CAD build for the part. Positions are in the model's coordinates, mm. Face numbers are marked on the shaded views. A direction names the side the tool comes from. Round coordinates to 2 decimals unless told otherwise and drop trailing zeros. Order: outer loops, then holes, each group sorted by start corner. A loop starts at its lowest first (then second) coordinate and runs counter-clockwise, first axis right, second up. Notation, with made-up numbers: M 31,7 L 48,7 A11 cw 48,14 Z; hole C -30,43.5 d7. An arc over 180 degrees is marked long. Answer as a JSON object with one key per item and string values.
```python
from build123d import *

# Parameters (mm, degrees)
CORTAR_EXTRUIR1_DEPTH = 9
CROQUIS5_R            = 4
CORTAR_EXTRUIR3_DEPTH = 27
CROQUIS6_R            = 2
CORTAR_EXTRUIR4_DEPTH = 10


with BuildPart() as part:
    # Croquis1 → Revolución1 (revolve)
    with BuildSketch(Plane(origin=(0, 0, 0), x_dir=(1, 0, 0), z_dir=(0, 1, 0))):
        Polygon((0, 1.5), (0, -9.5), (7, -9.5), (7, -13), (12.5, -13), (27.5, -13), (27.5, -7.5), (20, -7.5), (20, -2.5), (27.5, -2.5), (27.5, 2.5), (20, 2.5), (20, 7.5), (27.5, 7.5), (27.5, 13), (12.5, 13), (12.5, 6.5), (7.5, 1.5), align=None)
    revolve(axis=Axis((0, 0, 0), (0, 0, -1)))

    # Croquis2 → Cortar-Extruir1 (cut)
    with BuildSketch(Plane(origin=(0, 0, -1.5), x_dir=(-1, 0, 0), z_dir=(0, 0, -1))):
        Polygon((7.505553499, 0), (3.75277675, 6.5), (-3.75277675, 6.5), (-7.505553499, 0), (-3.75277675, -6.5), (3.75277675, -6.5), align=None)
    extrude(amount=-CORTAR_EXTRUIR1_DEPTH, mode=Mode.SUBTRACT)

    # Croquis5 → Cortar-Extruir3 (cut, through all)
    with BuildSketch(Plane.XY.offset(13)):
        with Locations((0, 24.5)):
            Circle(CROQUIS5_R)
        with Locations((12.25, 21.217622393)):
            Circle(CROQUIS5_R)
        with Locations((21.217622393, 12.25)):
            Circle(CROQUIS5_R)
        with Locations((24.5, 0)):
            Circle(CROQUIS5_R)
        with Locations((21.217622393, -12.25)):
            Circle(CROQUIS5_R)
        with Locations((12.25, -21.217622393)):
            Circle(CROQUIS5_R)
        with Locations((0, -24.5)):
            Circle(CROQUIS5_R)
        with Locations((-12.25, -21.217622393)):
            Circle(CROQUIS5_R)
        with Locations((-21.217622393, -12.25)):
            Circle(CROQUIS5_R)
        with Locations((-24.5, 0)):
            Circle(CROQUIS5_R)
        with Locations((-21.217622393, 12.25)):
            Circle(CROQUIS5_R)
        with Locations((-12.25, 21.217622393)):
            Circle(CROQUIS5_R)
    extrude(amount=-CORTAR_EXTRUIR3_DEPTH, mode=Mode.SUBTRACT)

    # Croquis6 → Cortar-Extruir4 (cut)
    with BuildSketch(Plane(origin=(0, 0, 7.5), x_dir=(-1, 0, 0), z_dir=(0, 0, -1))):
        Circle(CROQUIS6_R)
    extrude(amount=-CORTAR_EXTRUIR4_DEPTH, mode=Mode.SUBTRACT)


solid = part.part
```
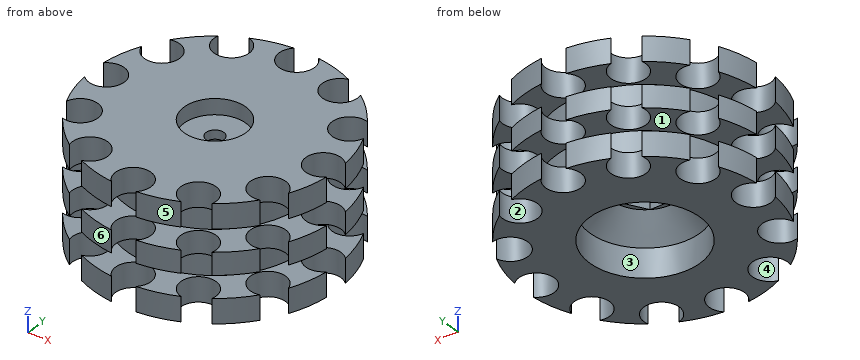
Item 1: Drop flat-ended pins along their axis: pin 1 Ø1.9 at (x, y) = (4.5, -2) entering from -Z; pin 2 Ø10 at (y, z) = (16.5, 5) entering from -X; pin 3 Ø6.5 at (x, y) = (-21.22, 12.25) entering from -Z; pin 4 Ø12 at (y, z) = (6.5, 5.5) entering from +X. Give the stop position or say it passes through.
Worked answers:
{"pin 1": "stops at z = 7.5", "pin 2": "stops at x = -22.29", "pin 3": "passes through", "pin 4": "stops at x = 27.36"}
Item 2: Two-plate mould, pull along X, no slides. Class the marked faces 4, 5 and 6: released by +X, released by -X, zero draft, split by the parting line, or undercut.
Worked answers:
{"face 4": "undercut", "face 5": "released by +X", "face 6": "released by -X"}
Item 3: Wall check: line 1 along Z through (x, y) = (-5, 21); line 2 along X through (y, z) = (-12, 8.25); line 3 along Y through (x, z) = (1, 0.75). Give the ranges that are in metal, low to high. Write a range as [from, to].
Worked answers:
{"line 1": "z = [-13, -7.5], [-2.5, 2.5], [7.5, 13]", "line 2": "x = [-17.23, 17.23]", "line 3": "y = [-20.63, -6.5], [6.5, 20.63]"}
Item 4: Saw through at B-B on y = 18. State how many separate pieces and enclosed holes the cut face has, and give its area (3 significant figures).
Worked answers:
{"separate pieces": "7", "enclosed holes": "0", "area": "688 mm2"}
Item 5: 3-axis set-ups, long thin cutter, end or side, ignore diameter. For the marked faces 1, 2 and 3: which of +Z, -Z, +X, -X, +Y, -Y reach the whole face in a straight line?
Worked answers:
{"face 1": "none", "face 2": "+Z, -Z", "face 3": "-Z"}
Item 6: Saw through at A-A on z = 6.5. List the corners of the cut face in (x, y), and give its area (3 significant figures).
Worked answers:
{"outline": "C 0,0 d40; hole M -7.51,0 L -3.75,-6.5 L 3.75,-6.5 L 7.51,0 L 3.75,6.5 L -3.75,6.5 Z", "area": "1,110 mm2"}
